from build123d import *

# Parameters (mm, degrees)
BOSS_EXTRUDE1_DEPTH      = 31
BOSS_EXTRUDE1_DEPTH_BACK = 32.5
SKETCH1_W                = 35
SKETCH1_H                = 60
FILLET2_RADIUS           = 17.5
FILLET2_LENGTH           = 63.5
BOSS_EXTRUDE2_DEPTH      = 32.5
BOSS_EXTRUDE2_DEPTH_BACK = 32.5
SKETCH8_W                = 35
SKETCH8_H                = 54
HOLE2_D                  = 20
CUT_EXTRUDE1_START       = -5
CUT_EXTRUDE1_DEPTH       = 5
CUT_EXTRUDE2_DEPTH       = 78.38539914
HOLE3_D                  = 20


with BuildPart() as part:
    # Sketch1 → Boss-Extrude1 (new, two sides: drawn at the far end of the back side and taken through both)
    with BuildSketch(Plane(origin=(0, 0, 0), x_dir=(0, 0, -1), z_dir=(1, 0, 0)).offset(-BOSS_EXTRUDE1_DEPTH_BACK)):
        Rectangle(SKETCH1_W, SKETCH1_H)
    extrude(amount=BOSS_EXTRUDE1_DEPTH + BOSS_EXTRUDE1_DEPTH_BACK)

    # Fillet2: full round fillet: the end face becomes a half cylinder, R = half its width
    fillet2_face = Plane((-0.75, 30, 0), x_dir=(1, 0, 0), z_dir=(0, 1, 0))  # on the end face: x along it, z out of the body
    fillet2_slab = fillet2_face.offset(-FILLET2_RADIUS / 2) * Box(FILLET2_LENGTH, 2 * FILLET2_RADIUS, FILLET2_RADIUS, mode=Mode.PRIVATE)  # the body's end, R deep
    fillet2_round = Plane((-0.75, 12.5, 0), x_dir=(0, 1, 0), z_dir=(1, 0, 0)) * Cylinder(FILLET2_RADIUS, FILLET2_LENGTH, mode=Mode.PRIVATE)  # its axis R under the face
    add(fillet2_slab - fillet2_round, mode=Mode.SUBTRACT)

    # Sketch8 → Boss-Extrude2 (add, two sides: drawn at the far end of the back side and taken through both)
    with BuildSketch(Plane.XY.offset(-BOSS_EXTRUDE2_DEPTH_BACK)):
        with Locations((0, -3)):
            Rectangle(SKETCH8_W, SKETCH8_H)
    extrude(amount=BOSS_EXTRUDE2_DEPTH + BOSS_EXTRUDE2_DEPTH_BACK)

    # Hole2 (through all)
    with Locations(Plane.XY.offset(32.5)):
        with Locations((0, 10)):
            Hole(HOLE2_D / 2)

    # Sketch14 → Cut-Extrude1 (cut)
    with BuildSketch(Plane.XY.offset(32.5).offset(CUT_EXTRUDE1_START)):
        with BuildLine():
            Line((-8.342416793, 4.486010332), (-11.877950699, 0.950476426))
            Line((-11.877950699, 0.950476426), (-9.049523574, -1.877950699))
            Line((-9.049523574, -1.877950699), (-5.513989668, 1.657583207))
            ThreePointArc((-5.513989668, 1.657583207), (-7.071067812, 2.928932188), (-8.342416793, 4.486010332))
        make_face()
    extrude(amount=CUT_EXTRUDE1_DEPTH, mode=Mode.SUBTRACT)

    # Sketch15 → Cut-Extrude2 (cut, through all)
    with BuildSketch(Plane(origin=(31, 0, 0), x_dir=(0, 0, -1), z_dir=(1, 0, 0))):
        Polygon((-12, -30), (-14.274437874, -23), (14.274437874, -23), (12, -30), align=None)
    extrude(amount=-CUT_EXTRUDE2_DEPTH, mode=Mode.SUBTRACT)

    # Hole3 (through all)
    with Locations(Plane(origin=(31, 0, 0), x_dir=(0, 0, -1), z_dir=(1, 0, 0))):
        with Locations((0, 12.5)):
            Hole(HOLE3_D / 2)


solid = part.part
The model under review builds one solid part; all positions refer to its coordinate system, in mm. A direction names the side the tool comes from. Round coordinates to 2 decimals unless told otherwise and drop trailing zeros. Loops run counter-clockwise (first coordinate to the right, second up) from the corner with the lowest first, then second, coordinate; pieces in that order, holes last. Notation, with made-up numbers: M 41,50.25 L 63,50.25 A22 ccw 63,68.25 Z; hole C 50.5,-4.5 d2. An arc over 180 degrees is marked long. Answer as CSV lines item,"result".
1. We need section A-A (x = 20.5). Give the boundary of the cut face in (y, z).
Outcome:
outline,"M -30,-17.5 L 12.5,-17.5 A17.5 ccw 12.5,17.5 L -30,17.5 L -30,12 L -23,14.27 L -23,-14.27 L -30,-12 Z; hole C 12.5,0 d20"
2. To check wall thickness, follow L1, parallel to Y at x = -10, z = 0; L2, parallel to Z at x = -17, y = 12.5; L3, parallel to Y at x = 0, z = 16. State the ranges of each line that lie inside material, in increasing order. Write a range as [from, to].
Outcome:
L1,"y = [-23, 2.5], [22.5, 30]"
L2,"z = [-32.5, -10], [10, 32.5]"
L3,"y = [-30, 0], [20, 24]"
3. For faces 5 (the face through (-25, -9, 17.5)), 6 (the face through (0, -23, 0)), 7 (the face through (24, -9, -17.5)), list the 3-axis set-ups (+Z, -Z, +X, -X, +Y, -Y) from which the entire face can be reached by the end or side of a thin tool; tool diameter is ignored.
Outcome:
face 5,"+Z, -X, +Y, -Y"
face 6,"+X, -X"
face 7,"-Z, +X, +Y, -Y"
4. We need section C-C (y = 10). Give the boundary of the cut face in (x, z).
Outcome:
outline,"M -32.5,-17.5 L -17.5,-17.5 L -17.5,-32.5 L -10,-32.5 L -10,-9.68 L -32.5,-9.68 Z; M -32.5,9.68 L -10,9.68 L -10,32.5 L -17.5,32.5 L -17.5,17.5 L -32.5,17.5 Z; M 10,-32.5 L 17.5,-32.5 L 17.5,-17.5 L 31,-17.5 L 31,-9.68 L 10,-9.68 Z; M 10,9.68 L 31,9.68 L 31,17.5 L 17.5,17.5 L 17.5,32.5 L 10,32.5 Z"
5. We need section B-B (z = -16.5). Give the boundary of the cut face in (x, y).
Outcome:
outline,"M -32.5,-30 L 31,-30 L 31,18.33 L 17.5,18.33 L 17.5,24 L -17.5,24 L -17.5,18.33 L -32.5,18.33 Z; hole C 0,10 d20"
6. Draft analysis for pull direction Y (two halves, no side actions). For faces 1 (the face through (-1, -30, -20)), 2 (the face through (-17.5, -3, 25)), 3 (the face through (-7.307, -0.135, 29.965)), 4 (the face through (2.17, 0.24, -0.45)), state which applies: pulls with the +Y half, pulls with the -Y half, needs draft (parallel to the pull), parting line crosses it, or undercut.
Outcome:
face 1,"pulls with the -Y half"
face 2,"needs draft"
face 3,"undercut"
face 4,"undercut"
7. Insertion check: pin 1 Ø9.5 at (x, z) = (-8, -21) entering from +Y; pin 2 Ø23 at (x, y) = (0, 10) entering from -Z; pin 3 Ø12 at (x, y) = (-28.5, -17.5) entering from +Z; pin 4 Ø15.5 at (y, z) = (1.5, -27) entering from -X. Each pin has a flat end and moves straight along its axis. Give the tip position at first contact, or say it passes through.
Outcome:
pin 1,"stops at y = 24"
pin 2,"stops at z = -32.5"
pin 3,"stops at z = 17.5"
pin 4,"stops at x = -17.5"
8. We need section D-D (x = 0). Give the boundary of the cut face in (y, z), plus the area to 3 significant figures.
Outcome:
outline,"M -30,-32.5 L 0,-32.5 L 0,32.5 L -30,32.5 L -30,12 L -23,14.27 L -23,-14.27 L -30,-12 Z; M 20,-32.5 L 24,-32.5 L 24,-13.19 A17.5 ccw 24,13.19 L 24,32.5 L 20,32.5 L 20,6.61 A10 cw 20,-6.61 Z"
area,"2,110 mm2"
